Geometry: see drawing. Coordinates: mm, zero at the bounding-box minimum. A direction names the side the tool comes from. Round coordinates to 2 decimals unless told otherwise and drop trailing zeros. Loops run counter-clockwise (first coordinate to the right, second up) from the corner with the lowest first, then second, coordinate; pieces in that order, holes last. Notation, with made-up numbers: (37.25, 62.25) - (86.25, 62.25) arc R10 ccw to (86.25, 67.25) - close; hole circle Ø1 at (64.25, -12). An arc over 180 degrees is marked (long way). Use CSV: the item, a comma, the result in double quotes. Start each with the question number.
1. Cut plane B-B (y = 26.5). Return loops of the section in (x, z) (1 decimal).
2. Cut plane A-A (z = 6.5). Return loops of the section in (x, y) (1 decimal).
3. Pin query (flat end, axial travel): P1, Ø6, axis at x = 24, y = 35, coming from the -Z side; P2, Ø1, axis at x = 2, z = 1, coming from the +Y side (1 decimal); P3, Ø2.5, axis at x = 14, y = 3.5, coming from the -Z side. Return the tip coordinate at first contact, or that it passes through.
4. Access query for the marked faces 1 and 2. Directions: +Z, -Z, +X, -X, +Y, -Y. A direction counts if a zero-diameter tool reaches every point of the face in a straight line with its end or side. Return the directions, or none.
5. Cut plane C-C (x = 10). Return loops of the section in (y, z) (1 decimal).
6. Pull-direction query (Y, two-part tool) for the marked faces 3, 4 and 5; classes: +Y half, -Y half, draft (parallel to the pull), parting line (faces both ways), or undercut.
7. Material intervals for probe 1 along X at (y, z) = (4, 13.25) (1 decimal); probe 2 along X at (y, z) = (47, 11.25) (1 decimal); probe 3 along Y at (x, z) = (14, 12.5), sorted ascending. Write a range as from..to.
8. Cut plane D-D (z = 2.75). Return loops of the section in (x, y) (1 decimal).
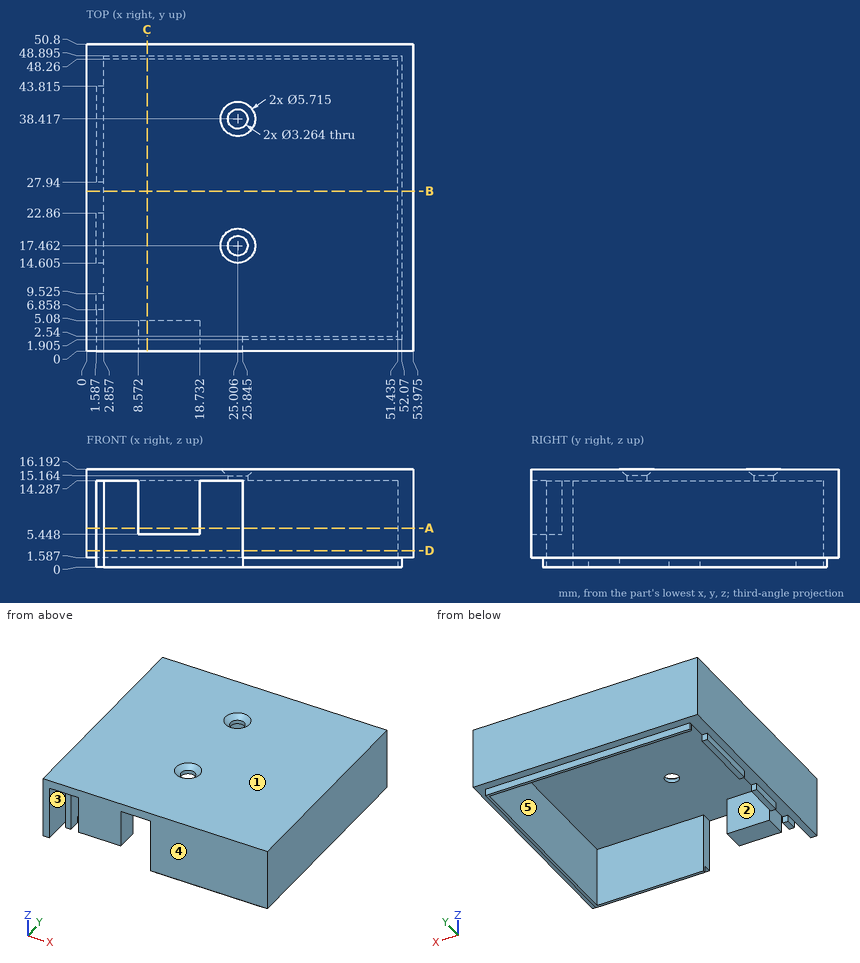
Established:
1,outline,"(0, 1.6) - (2.9, 1.6) - (2.9, 14.3) - (51.4, 14.3) - (51.4, 0) - (52.1, 0) - (52.1, 1.6) - (54, 1.6) - (54, 16.2) - (0, 16.2) - close"
2,outline,"(0, 0) - (1.6, 0) - (1.6, 6.9) - (2.9, 6.9) - (2.9, 48.3) - (51.4, 48.3) - (51.4, 2.5) - (25.8, 2.5) - (25.8, 0) - (54, 0) - (54, 50.8) - (0, 50.8) - close; (8.6, 0) - (18.7, 0) - (18.7, 5.1) - (8.6, 5.1) - close"
3,P1,"stops at z = 14.29"
3,P2,"stops at y = 43.8"
3,P3,"stops at z = 5.45"
4,face 1,"+Z, +X, -X, +Y, -Y"
4,face 2,"-Z"
5,outline,"(0, 5.4) - (5.1, 5.4) - (5.1, 14.3) - (48.3, 14.3) - (48.3, 0) - (48.9, 0) - (48.9, 1.6) - (50.8, 1.6) - (50.8, 16.2) - (0, 16.2) - close"
6,face 3,"draft"
6,face 4,"-Y half"
6,face 5,"undercut"
7,probe 1,"x = 0..1.6, 8.6..18.7, 51.4..54"
7,probe 2,"x = 0..2.9, 51.4..54"
7,probe 3,"y = 0..5.08, 48.26..50.8"
8,outline,"(0, 0) - (1.6, 0) - (1.6, 6.9) - (2.9, 6.9) - (2.9, 48.3) - (51.4, 48.3) - (51.4, 2.5) - (25.8, 2.5) - (25.8, 0) - (54, 0) - (54, 50.8) - (0, 50.8) - close"
